```python
from build123d import *

# Parameters (mm, degrees)
SKETCH1_R           = 17.5
SKETCH1_R_2         = 6
BOSS_EXTRUDE1_DEPTH = 15
SKETCH2_R           = 2.25
CUT_EXTRUDE1_DEPTH  = 29.939592257
SKETCH3_R           = 1.25
CUT_EXTRUDE2_DEPTH  = 29.93959243


with BuildPart() as part:
    # Sketch1 → Boss-Extrude1 (new body)
    with BuildSketch(Plane.XY):
        Circle(SKETCH1_R)
        Circle(SKETCH1_R_2, mode=Mode.SUBTRACT)
    extrude(amount=BOSS_EXTRUDE1_DEPTH)

    # Sketch2 → Cut-Extrude1 (cut, through all)
    with BuildSketch(Plane(origin=(0, 0, 0), x_dir=(1, 0, 0), z_dir=(0, 1, 0))):
        with Locations(Location((0, -7.5, 0), (0, 0, 270))):
            Circle(SKETCH2_R)
    extrude(amount=-CUT_EXTRUDE1_DEPTH, mode=Mode.SUBTRACT)

    # Sketch3 → Cut-Extrude2 (cut, through all)
    with BuildSketch(Plane.XY.offset(15)):
        with Locations((0, 12.5)):
            Circle(SKETCH3_R)
        with Locations((10.825317547, -6.25)):
            Circle(SKETCH3_R)
        with Locations((-10.825317547, -6.25)):
            Circle(SKETCH3_R)
    extrude(amount=-CUT_EXTRUDE2_DEPTH, mode=Mode.SUBTRACT)


solid = part.part
```
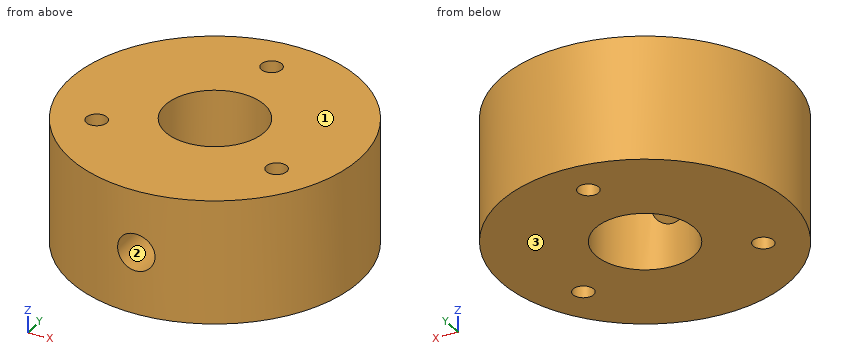
CAD build for the part. Positions are in the model's coordinates, mm. Face numbers are marked on the shaded views. Give positions to 0.01 mm unless a question says otherwise; leave off trailing zeros. Loops run counter-clockwise (first coordinate to the right, second up) from the corner with the lowest first, then second, coordinate; pieces in that order, holes last. Notation, with made-up numbers: (77.25, -11.75) - (81.25, -11.75) arc R10 ccw to (81.25, 7.25) - close; hole circle Ø2 at (56, 84.25). An arc over 180 degrees is marked (long way). Put each result on its own line as item: value.
Q1. Slice it at D-D (y = -10.5). Give the cut face in (x, z), plus the area to 3 significant figures.
Filled in:
outline: (-14, 0) - (14, 0) - (14, 15) - (-14, 15) - close; hole circle Ø4.5 at (0, 7.5)
area: 404 mm²
Q2. Flat gauge pins, fed straight in: pin 1 (3 mm diameter, centred on x = -10.83, y = -6.25, fed in from -Z); pin 2 (1 mm diameter, centred on x = -11.5, z = 12.5, fed in from -Y); pin 3 (3 mm diameter, centred on y = 7.5, z = 12, fed in from +X); pin 4 (5 mm diameter, centred on y = -6.5, z = 8.5, fed in from -X). Where does each tip first touch, or does it go through?
Filled in:
pin 1: stops at z = 0
pin 2: stops at y = -13.61
pin 3: stops at x = 16.44
pin 4: stops at x = -17.04
Q3. Mould opens along Z. For the marked faces 1, 2 and 3 say: pulls with the +Z half, pulls with the -Z half, needs draft (parallel to the pull), parting line crosses it, or undercut.
Filled in:
face 1: pulls with the +Z half
face 2: undercut
face 3: pulls with the -Z half
Q4. Slice it at B-B (x = 0). Give the cut face in (y, z), plus the area to 3 significant figures.
Filled in:
outline: (-17.5, 0) - (-6, 0) - (-6, 5.25) - (-17.5, 5.25) - close; (-17.5, 9.75) - (-6, 9.75) - (-6, 15) - (-17.5, 15) - close; (6, 0) - (11.25, 0) - (11.25, 15) - (6, 15) - close; (13.75, 0) - (17.5, 0) - (17.5, 15) - (13.75, 15) - close
area: 256 mm²
Q5. Probe line 1 along Z through (x, y) = (0, -13.5); line 2 along Y through (x, z) = (1, 2.25); line 3 along Y through (x, z) = (0, 5.5). List the from-to ranges inside material, lowest first.
Filled in:
line 1: z = 0 to 5.25, 9.75 to 15
line 2: y = -17.47 to -5.92, 5.92 to 11.75, 13.25 to 17.47
line 3: y = 6 to 11.25, 13.75 to 17.5
Q6. Slice it at C-C (z = 12.5). Give the cut face in (x, y), plus the area to 3 significant figures.
Filled in:
outline: circle Ø35 at (0, 0); hole circle Ø2.5 at (-10.83, -6.25); hole circle Ø12 at (0, 0); hole circle Ø2.5 at (0, 12.5); hole circle Ø2.5 at (10.83, -6.25)
area: 834 mm²
Q7. Slice it at A-A (y = 0). Give the cut face in (x, z).
Filled in:
outline: (-17.5, 0) - (-6, 0) - (-6, 15) - (-17.5, 15) - close; (6, 0) - (17.5, 0) - (17.5, 15) - (6, 15) - close
